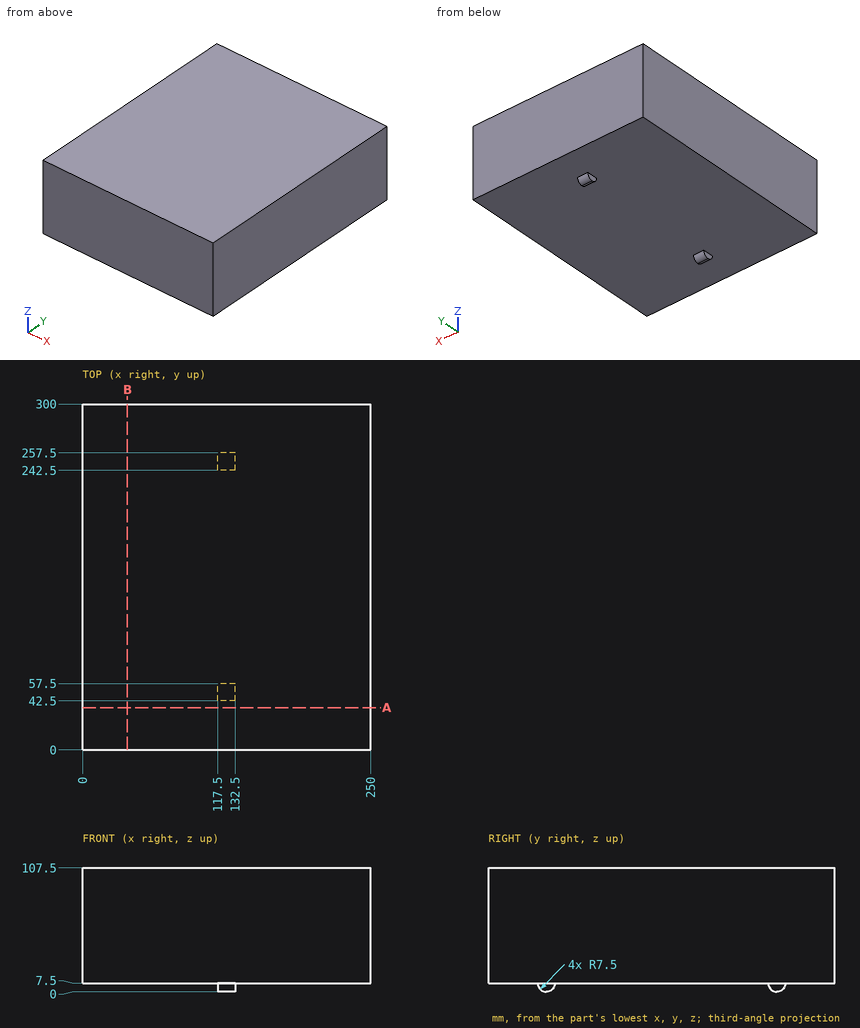
Geometry: see drawing. Coordinates: mm, zero at the bounding-box minimum. Coordinates: 2 decimals unless noted, no trailing zeros. Order: outer loops, then holes, each group sorted by start corner. A loop starts at its lowest first (then second) coordinate and runs counter-clockwise, first axis right, second up. Notation, with made-up numbers: M 38.25,5.5 L 51.25,5.5 A14 ccw 51.25,32.5 Z; hole C 34.25,-20 d2. An arc over 180 degrees is marked long. Answer in a Markdown table with one row per item. Add a question column.
Q1. Contact query for flat-ended pins moving along their axis: P1, Ø4, axis at y = 50, z = 5, coming from the -X side; P2, Ø10, axis at x = 141.5, y = 93, coming from the -Z side; P3, Ø4, axis at y = 251, z = 2.5, coming from the +X side. Output: stop coordinate, or through.
Q2. Section query B-B on x = 39. Return the cut outline in (y, z).
Q3. Section query A-A on y = 36.5. Return the cut outline in (x, z).
Q4. Line query: L1, parallel to Z at x = 182, y = 103. Output: solid intervals per line, ascending.
Completed:
| question | item | result |
|---|---|---|
| 1 | P1 | stops at x = 117.5 |
| 1 | P2 | stops at z = 7.5 |
| 1 | P3 | stops at x = 132.5 |
| 2 | outline | M 0,7.5 L 300,7.5 L 300,107.5 L 0,107.5 Z |
| 3 | outline | M 0,7.5 L 250,7.5 L 250,107.5 L 0,107.5 Z |
| 4 | L1 | z = 7.5 to 107.5 |
